Source: CAD feature listing. Evaluate the final solid. Frame: model axes, mm. Coordinates: 2 decimals unless noted, no trailing zeros. Order: outer loops, then holes, each group sorted by start corner. A loop starts at its lowest first (then second) coordinate and runs counter-clockwise, first axis right, second up.
Item 1: Section A-A on y = 48.5. Return the cut outline in (x, z), then the cut area to 3 significant figures.
Item 2: Section C-C on y = 55. Return the cut outline in (x, z), then the cut area to 3 significant figures.
Item 3: Ray query, line 1 (X direction, y = 49, z = 2); line 2 (X direction, y = 52.5, z = 1); line 3 (Y direction, x = 48, z = 4.25). Return the intervals inside material, ascending.
Item 4: Contact query for flat-ended pins moving along their axis: P1, Ø1, axis at y = 49.5, z = 5, coming from the -X side; P2, Ø2, axis at y = 57.5, z = 3.5, coming from the +X side. Output: stop coordinate, or through.
Item 5: Section B-B on z = 1. Return the cut outline in (x, y) (3 decimals), then the cut area to 3 significant figures.
from build123d import *

# Parameters (mm, degrees)
F2_DEPTH = 6.35
F1_R     = 3.175
F3_DEPTH = 6.351


with BuildPart() as f2:
    # F0 (on Top) → F2 (new body)
    with BuildSketch(Plane.XY):
        with BuildLine():
            ThreePointArc((-37.093219, 60.618736), (-47.093219, 50.618736), (-37.093219, 40.618736))
            Line((-37.093219, 40.618736), (50.406781, 40.618736))
            ThreePointArc((50.406781, 40.618736), (60.406781, 50.618736), (50.406781, 60.618736))
            Line((50.406781, 60.618736), (-37.093219, 60.618736))
        make_face()
    extrude(amount=F2_DEPTH)

    # F1 (on face) → F3 (cut, through all)
    with BuildSketch(Plane.XY):
        with Locations((-37.093219, 50.618736)):
            Circle(F1_R)
        with Locations((50.406781, 50.618736)):
            Circle(F1_R)
        with Locations((1.756781, 50.618736)):
            Circle(F1_R)
    extrude(amount=F3_DEPTH, mode=Mode.SUBTRACT)


solid = f2.part
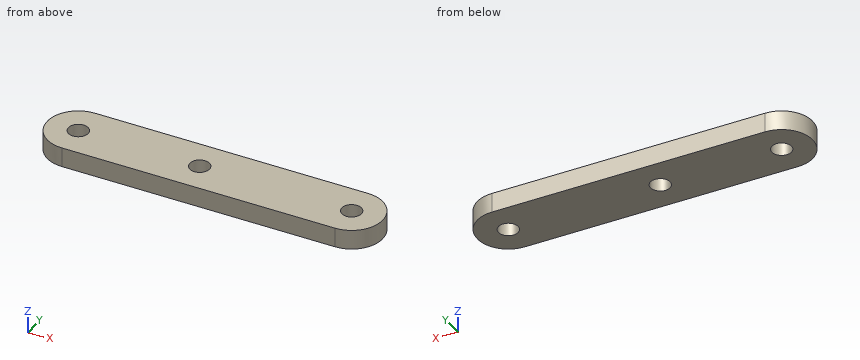
Answer list:
1. outline: (-46.87, 0) - (-39.46, 0) - (-39.46, 6.35) - (-46.87, 6.35) - close; (-34.73, 0) - (-0.61, 0) - (-0.61, 6.35) - (-34.73, 6.35) - close; (4.12, 0) - (48.04, 0) - (48.04, 6.35) - (4.12, 6.35) - close; (52.77, 0) - (60.18, 0) - (60.18, 6.35) - (52.77, 6.35) - close
1. area: 590 mm2
2. outline: (-46.08, 0) - (59.4, 0) - (59.4, 6.35) - (-46.08, 6.35) - close
2. area: 670 mm2
3. line 1: x = -46.96 to -39.82, -34.36 to -0.97, 4.49 to 47.68, 53.14 to 60.27
3. line 2: x = -46.91 to -39.65, -34.54 to -0.8, 4.31 to 47.85, 52.96 to 60.23
3. line 3: y = 40.62 to 48.55, 52.69 to 60.62
4. P1: stops at x = -47.07
4. P2: stops at x = 58.49
5. outline: (-37.093, 40.619) - (50.407, 40.619) arc R10 ccw to (50.407, 60.619) - (-37.093, 60.619) arc R10 ccw to start; hole circle Ø6.35 at (-37.093, 50.619); hole circle Ø6.35 at (1.757, 50.619); hole circle Ø6.35 at (50.407, 50.619)
5. area: 1,970 mm2
